Input: part model. Units: mm. Frame: model coordinates. Give positions to 0.01 mm unless a question says otherwise; leave off trailing zeros. Loops run counter-clockwise (first coordinate to the right, second up) from the corner with the lowest first, then second, coordinate; pieces in that order, holes last. Notation, with made-up numbers: M 10,62 L 57,62 A7 cw 57,71 Z; hole C -22,7.25 d7. An arc over 180 degrees is marked long. Return JSON: item names as keys, results as strings. Group by question number.
```python
from build123d import *

# Parameters (mm, degrees)
BOSS_EXTRUDE1_DEPTH = 468
SKETCH2_R           = 6
CUT_EXTRUDE1_DEPTH  = 3.175


with BuildPart() as part:
    # Sketch1 → Boss-Extrude1 (new body)
    with BuildSketch(Plane(origin=(0, 0, 0), x_dir=(0, 0, -1), z_dir=(1, 0, 0))):
        Polygon((0, 0), (0, 19.05), (3.175, 19.05), (3.175, 3.175), (19.05, 3.175), (19.05, 0), align=None)
    extrude(amount=-BOSS_EXTRUDE1_DEPTH)

    # Sketch2 → Cut-Extrude1 (cut)
    with BuildSketch(Plane.XY):
        with Locations((-450.13, 11.273546723)):
            Circle(SKETCH2_R)
        with Locations((-414.38, 11.273546723)):
            Circle(SKETCH2_R)
        with Locations((-378.63, 11.273546723)):
            Circle(SKETCH2_R)
        with Locations((-342.88, 11.273546723)):
            Circle(SKETCH2_R)
        with Locations((-307.13, 11.273546723)):
            Circle(SKETCH2_R)
        with Locations((-271.38, 11.273546723)):
            Circle(SKETCH2_R)
        with Locations((-235.63, 11.273546723)):
            Circle(SKETCH2_R)
        with Locations((-199.88, 11.273546723)):
            Circle(SKETCH2_R)
        with Locations((-164.13, 11.273546723)):
            Circle(SKETCH2_R)
        with Locations((-128.38, 11.273546723)):
            Circle(SKETCH2_R)
        with Locations((-92.63, 11.273546723)):
            Circle(SKETCH2_R)
        with Locations((-56.88, 11.273546723)):
            Circle(SKETCH2_R)
        with Locations((-21.13, 11.273546723)):
            Circle(SKETCH2_R)
    extrude(amount=-CUT_EXTRUDE1_DEPTH, mode=Mode.SUBTRACT)


solid = part.part
```
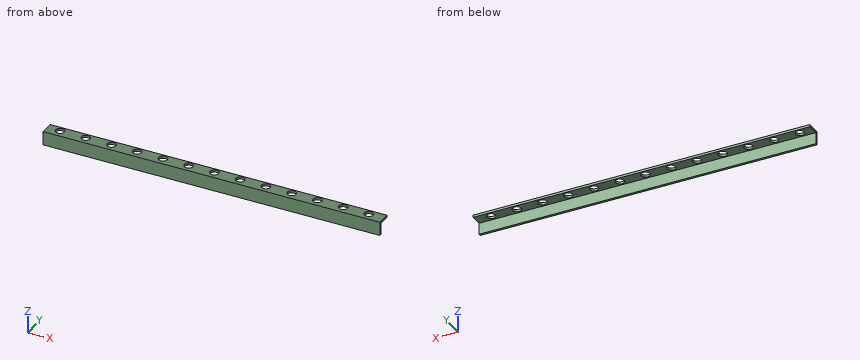
Item 1: Section B-B, the plane x = -187. Return loops of the section in (y, z) (3 decimals).
Item 2: Section C-C, the plane x = -94. Return loops of the section in (y, z) (3 decimals), then the cut area to 3 significant figures.
Item 3: Material intervals for line 1 (Y direction, x = -164.13, z = -0.95); line 2 (Z direction, x = -206, y = 6) (3 decimals); line 3 (Y direction, x = -281, z = -13.5) (3 decimals), sorted ascending. Write a range as from..to.
Item 4: Section D-D, the plane z = -11. Return loops of the section in (x, y) (3 decimals), then the cut area to 3 significant figures.
Item 5: First-contact query: pin 1 Ø11 at (x, y) = (-128.38, 11.27) entering from +Z. Flat tip, straight axial feed; report the tip coordinate or a pass-through.
Item 6: Section A-A, the plane x = -307.13. Return loops of the section in (y, z) (3 decimals).
Answer below:
{
 "1": {"outline": "M 0,-19.05 L 3.175,-19.05 L 3.175,-3.175 L 19.05,-3.175 L 19.05,0 L 0,0 Z"},
 "2": {"outline": "M 0,-19.05 L 3.175,-19.05 L 3.175,-3.175 L 5.432,-3.175 L 5.432,0 L 0,0 Z; M 17.115,-3.175 L 19.05,-3.175 L 19.05,0 L 17.115,0 Z", "area": "73.8 mm^2"},
 "3": {"line 1": "0..5.27, 17.27..19.05", "line 2": "-3.175..0", "line 3": "0..3.175"},
 "4": {"outline": "M -468,0 L 0,0 L 0,3.175 L -468,3.175 Z", "area": "1,490 mm^2"},
 "5": {"pin 1": "through"},
 "6": {"outline": "M 0,-19.05 L 3.175,-19.05 L 3.175,-3.175 L 5.274,-3.175 L 5.274,0 L 0,0 Z; M 17.274,-3.175 L 19.05,-3.175 L 19.05,0 L 17.274,0 Z"}
}
